Design review of the part built by this model. Coordinates are the model's own, in mm. A direction names the side the tool comes from. Coordinates: 2 decimals unless noted, no trailing zeros. Loops run counter-clockwise (first coordinate to the right, second up) from the corner with the lowest first, then second, coordinate; pieces in that order, holes last.
from build123d import *

# Parameters (mm, degrees)
BOSS_EXTRUDE1_DEPTH             = 50
CUT_EXTRUDE1_DEPTH              = 76.498344353
SKETCH5_W                       = 25
SKETCH5_H                       = 50
BOSS_EXTRUDE2_DEPTH             = 30
F_20_5_20_5_DIAMETER_HOLE1_D    = 20.5
F_5_7_5_7_DIAMETER_HOLE1_REACH  = 130.282
F_5_7_5_7_DIAMETER_HOLE1_BORE_R = 2.85
F_5_7_5_7_DIAMETER_HOLE2_D      = 5.7
F_5_7_5_7_DIAMETER_HOLE2_DEPTH  = 11.568542495
F_5_7_5_7_DIAMETER_HOLE2_TIP    = 1.712452764


with BuildPart() as part:
    # Sketch2 → Boss-Extrude1 (new body)
    with BuildSketch(Plane(origin=(0, 0, 0), x_dir=(1, 0, 0), z_dir=(0, 1, 0))):
        Polygon((-40, -40), (40, 40), (40, -40), align=None)
    extrude(amount=BOSS_EXTRUDE1_DEPTH)

    # Sketch4 → Cut-Extrude1 (cut, through all)
    with BuildSketch(Plane(origin=(0, 50, 0), x_dir=(1, 0, 0), z_dir=(0, 1, 0))):
        Polygon((17.67766953, 17.67766953), (-17.67766953, -17.67766953), (-3.535533906, -31.819805153), (31.819805153, 3.535533906), align=None)
        Polygon((31.819805153, 31.819805153), (17.67766953, 17.67766953), (31.819805153, 3.535533906), align=None)
        Polygon((-17.67766953, -17.67766953), (-31.819805153, -31.819805153), (-3.535533906, -31.819805153), align=None)
        Polygon((40, -4.644660941), (4.644660941, -40), (40, -40), align=None)
    extrude(amount=-CUT_EXTRUDE1_DEPTH, mode=Mode.SUBTRACT)

    # Sketch5 → Boss-Extrude2 (add)
    with BuildSketch(Plane(origin=(22.32233047, 0, 22.32233047), x_dir=(0.7071067811865474, 0, -0.7071067811865477), z_dir=(0.7071067811865477, 0, 0.7071067811865474))):
        with Locations((0, 25)):
            Rectangle(SKETCH5_W, SKETCH5_H)
    extrude(amount=BOSS_EXTRUDE2_DEPTH)

    # Ø20.5 (20.5) Diameter Hole1 (through all)
    with Locations(Plane(origin=(0, 50, 0), x_dir=(1, 0, 0), z_dir=(0, 1, 0))):
        with Locations((32.928932188, -32.928932188)):
            Hole(F_20_5_20_5_DIAMETER_HOLE1_D / 2)

    # Ø5.7 (5.7) Diameter Hole1 bore → Ø5.7 (5.7) Diameter Hole1 (cut, up to next)
    with BuildSketch(Plane(origin=(43.535533906, 0, 43.535533906), x_dir=(0.7071067811865476, 0, -0.7071067811865476), z_dir=(0.7071067811865476, 0, 0.7071067811865476)), mode=Mode.PRIVATE) as f_5_7_5_7_diameter_hole1_sk1:
        with Locations((0, 25)):
            Circle(F_5_7_5_7_DIAMETER_HOLE1_BORE_R)
    f_5_7_5_7_diameter_hole1_tool1 = extrude(f_5_7_5_7_diameter_hole1_sk1.sketch, amount=-F_5_7_5_7_DIAMETER_HOLE1_REACH, mode=Mode.PRIVATE) & part.part
    add(f_5_7_5_7_diameter_hole1_tool1.solids().sort_by_distance((43.535534, 25, 43.535534))[0], mode=Mode.SUBTRACT)

    # Ø5.7 (5.7) Diameter Hole2
    with Locations(Plane(origin=(22.32233047, 0, 22.32233047), x_dir=(0.7071067811865474, 0, -0.7071067811865477), z_dir=(0.7071067811865477, 0, 0.7071067811865474))):
        with Locations((-18.75, 38.75), (18.75, 38.75), (18.75, 11.25), (-18.75, 11.25)):
            Hole(F_5_7_5_7_DIAMETER_HOLE2_D / 2, depth=F_5_7_5_7_DIAMETER_HOLE2_DEPTH)
            with Locations((0, 0, -(F_5_7_5_7_DIAMETER_HOLE2_DEPTH + F_5_7_5_7_DIAMETER_HOLE2_TIP / 2))):  # 118° drill point
                Cone(0, F_5_7_5_7_DIAMETER_HOLE2_D / 2, F_5_7_5_7_DIAMETER_HOLE2_TIP, mode=Mode.SUBTRACT)


solid = part.part
Q1. Take a section at C-C, the plane z = -20. Write out the cut boundary in (x, y), then the cut area to 3 significant figures.
Q2. For line 1 (X direction, y = 32.5, z = 34.5); line 2 (X direction, y = 48, z = 35.5); line 3 (Z direction, x = 32, y = 20), list the stretches that pass through material, from the lowest coordinate up.
Q3. The part is to be moulded in two halves that separate along X. For faces 1 (the flat face through (41.62, 24.65, 23.94)), 2 (the flat face through (13.895, 25.35, 14.39)), 3 (the cylindrical face through (23.152, 24.65, 29.85)), say which applies: pulls with the +X half, pulls with the -X half, needs draft (parallel to the pull), parting line crosses it, or undercut.
Q4. Machinability: for faces 4 (the flat face through (23.94, 24.65, 41.62)), 5 (the flat face through (-17, 25, 40)), 6 (the flat face through (-18, 25, 31.82)), which of the approach directions +Z, -Z, +X, -X, +Y, -Y give a long, thin tool a straight path to every point of the face, cutting with its end or side? Answer none if there is none.
Q5. Take a section at B-B, the plane y = 30.5. Write out the cut boundary in (x, z), then the cut area to 3 significant figures.
Q6. Take a section at A-A, the plane x = 24. Write out the cut boundary in (y, z).
Q7. Clearance check with flat-ended pins moving along their axes: pin 1 Ø4 at (x, y) = (5.5, 11.5) entering from +Z; pin 2 Ø22.5 at (y, z) = (25, -10) entering from +X; pin 3 Ø6 at (x, y) = (5.5, 11) entering from -Z. State where each tip first meets the part, or that it passes through.
Q8. Take a section at D-D, the plane x = -18.5. Write out the cut boundary in (y, z), then the cut area to 3 significant figures.
Entries:
1. outline: (31.82, 0) - (40, 0) - (40, 50) - (31.82, 50) - close
1. area: 409 mm2
2. line 1: x = -34.5 to 10.14, 16.82 to 22.8, 43.06 to 52.18
2. line 2: x = -35.5 to 9.14, 17.82 to 23.01, 42.85 to 51.57
2. line 3: z = -32 to 12.64, 14.32 to 22.72, 43.14 to 49.68
3. face 1: pulls with the +X half
3. face 2: pulls with the -X half
3. face 3: undercut
4. face 4: +Z, +Y, -Y
4. face 5: +Z, -X, +Y, -Y
4. face 6: -Z, -X, +Y, -Y
5. outline: (-40, 40) - (-31.82, 31.82) - (-3.54, 31.82) - (31.82, -3.54) - (31.82, -31.82) - (40, -40) - (40, 4.64) - (31.16, 13.48) - (52.37, 34.7) - (34.7, 52.37) - (13.48, 31.16) - (4.64, 40) - close; hole circle Ø20.5 at (32.93, 32.93)
5. area: 1,590 mm2
6. outline: (0, 4.28) - (50, 4.28) - (50, 27.9) - (0, 27.9) - close; (0, 37.96) - (50, 37.96) - (50, 41.68) - (0, 41.68) - close
7. pin 1: stops at z = 40
7. pin 2: stops at x = 40
7. pin 3: stops at z = 19.78
8. outline: (0, 31.82) - (50, 31.82) - (50, 40) - (0, 40) - close
8. area: 409 mm2
